Answer from the drawing. Dimensions are ordinates in mm from the lowest x, y and z of the part. A direction names the side the tool comes from. Give positions to 0.01 mm unless a question says otherwise; leave off trailing zeros. Write each loop counter-clockwise with the first axis right and the second up, starting at its lowest first coordinate (ties: lowest second). Pieces come first, ordered by that corner, then holes. Notation, with made-up numbers: (38.25, 64) -> (69.25, 64) arc R7 ccw to (69.25, 75) -> close; hole circle Ø10 at (51, 19). An arc over 180 degrees is marked (long way). Put each result on its own line as item: value. Start each with the question number.
1) For the marked faces 1 and 2, determine the directions among +Z, -Z, +X, -X, +Y, -Y from which every point of the face is accessible in a straight line to the end or side of a thin tool.
2) A cutting plane is placed at A-A (z = 4). Write down the section's boundary in (x, y).
3) A cutting plane is placed at B-B (z = 20.25). Write down the section's boundary in (x, y).
4) Find the intervals of material crossed by line 1 along Z through (x, y) = (2.5, 4.55); line 2 along Y through (x, z) = (2.5, 3.5); line 3 along X through (y, z) = (4, 15.75) (1 decimal), in increasing order. Write a range as from..to.
5) A cutting plane is placed at C-C (y = 4.55). Write down the section's boundary in (x, z).
6) A cutting plane is placed at D-D (x = 5.2). Write down the section's boundary in (y, z).
7) Flat-ended cylindrical pins translate along their axes: pin 1 Ø3 at (y, z) = (2, 21.5) entering from +X; pin 2 Ø2 at (x, y) = (2.89, 2.5) entering from -Z. Find the tip coordinate at first contact, or state that the pin passes through.
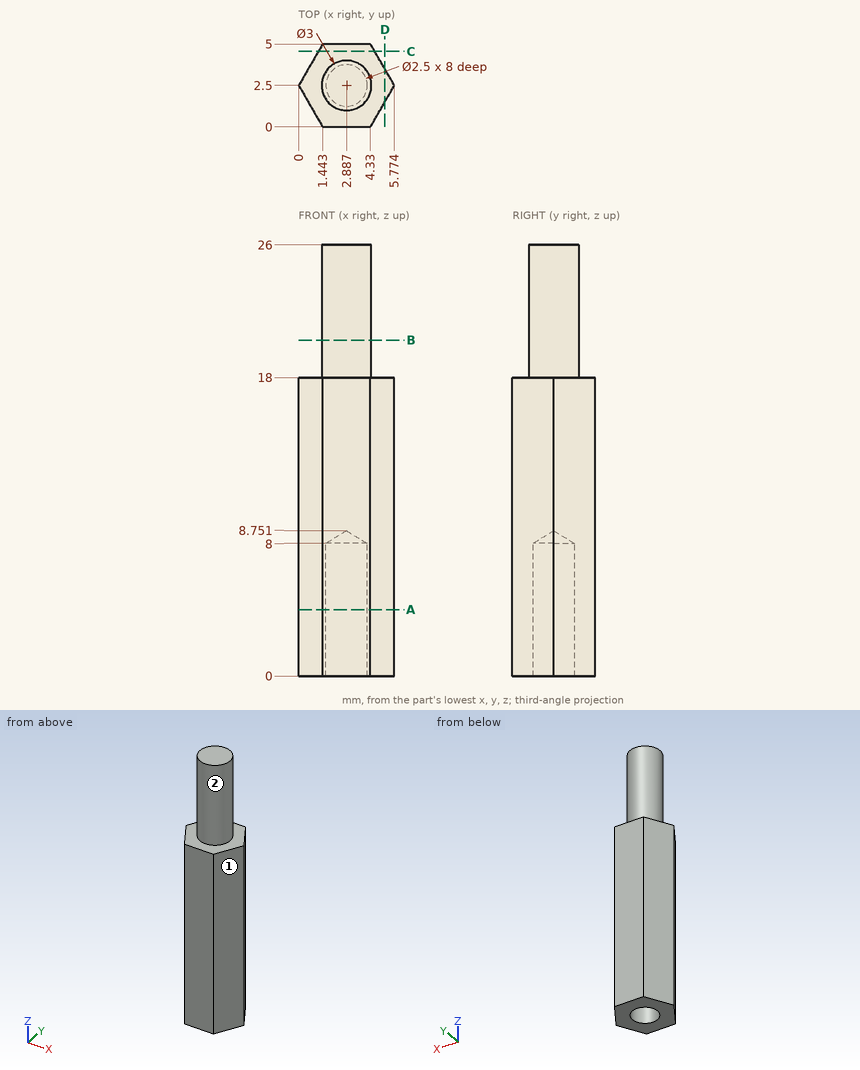
Reply:
1. face 1: +Z, -Z, +X, -Y
1. face 2: +Z
2. outline: (0, 2.5) -> (1.44, 0) -> (4.33, 0) -> (5.77, 2.5) -> (4.33, 5) -> (1.44, 5) -> close; hole circle Ø2.5 at (2.89, 2.5)
3. outline: circle Ø3 at (2.89, 2.5)
4. line 1: z = 0..18
4. line 2: y = 0..1.31, 3.69..5
4. line 3: x = 0.9..4.9
5. outline: (1.18, 0) -> (4.59, 0) -> (4.59, 18) -> (1.18, 18) -> close
6. outline: (1.51, 0) -> (3.49, 0) -> (3.49, 18) -> (1.51, 18) -> close
7. pin 1: stops at x = 4.39
7. pin 2: stops at z = 8.15
